from build123d import *

# Parameters (mm, degrees)
SKETCH1_W              = 16.002
SKETCH1_H              = 36.576
BOSS_EXTRUDE1_DEPTH    = 7.112
BOSS_EXTRUDE2_DEPTH    = 6.604
SKETCH3_W              = 16.002
SKETCH3_H              = 6.604
CUT_EXTRUDE1_DEPTH     = 2.54
SKETCH4_W              = 16.002
SKETCH4_H              = 2.54
CUT_EXTRUDE2_DEPTH     = 6.604
BOSS_EXTRUDE3_DEPTH    = 32.004
SKETCH6_W              = 32.004
SKETCH6_H              = 36.576
BOSS_EXTRUDE4_DEPTH    = 2.032
SKETCH7_W              = 16.002
SKETCH7_H              = 2.54
CUT_EXTRUDE3_DEPTH     = 6.604
M3_5_CLEARANCE_HOLE1_D = 3.7973


with BuildPart() as part:
    # Sketch1 → Boss-Extrude1 (new body)
    with BuildSketch(Plane(origin=(0, 7.874, 0), x_dir=(1, 0, 0), z_dir=(0, 1, 0))):
        with Locations((-8.001, 0)):
            Rectangle(SKETCH1_W, SKETCH1_H)
    extrude(amount=-BOSS_EXTRUDE1_DEPTH)

    # Sketch2 → Boss-Extrude2 (add)
    with BuildSketch(Plane.XZ.offset(-0.762)):
        with BuildLine():
            Line((-16.002, -18.288), (-16.002, 18.288))
            Line((-16.002, 18.288), (0, 18.288))
            Line((0, 18.288), (0, -15.748))
            add(Edge.make_bspline(
                [(0, -18.288), (0, -17.441333333), (0, -16.594666667), (0, -15.748)],
                knots=[0, 0, 0, 0, 1, 1, 1, 1], degree=3))
            Line((0, -18.288), (-16.002, -18.288))
        make_face()
    extrude(amount=BOSS_EXTRUDE2_DEPTH)

    # Sketch3 → Cut-Extrude1 (cut)
    with BuildSketch(Plane(origin=(0, 0, -18.288), x_dir=(-1, 0, 0), z_dir=(0, 0, -1))):
        with Locations((8.001, -2.54)):
            Rectangle(SKETCH3_W, SKETCH3_H)
    extrude(amount=-CUT_EXTRUDE1_DEPTH, mode=Mode.SUBTRACT)

    # Sketch4 → Cut-Extrude2 (cut)
    with BuildSketch(Plane.XZ.offset(5.842)):
        with Locations((-8.001, 17.018)):
            Rectangle(SKETCH4_W, SKETCH4_H)
    extrude(amount=-CUT_EXTRUDE2_DEPTH, mode=Mode.SUBTRACT)

    # Sketch5 → Boss-Extrude3 (add)
    with BuildSketch(Plane(origin=(0, 0, 0), x_dir=(0, 0, -1), z_dir=(1, 0, 0))):
        with BuildLine():
            Line((-18.288, -5.842), (-18.288, 0))
            ThreePointArc((-18.288, 0), (-12.964507707, 7.449482293), (-4.192296053, 4.826))
            Line((-4.192296053, 4.826), (4.192296053, 4.826))
            ThreePointArc((4.192296053, 4.826), (12.964507707, 7.449482293), (18.288, 0))
            Line((18.288, 0), (18.288, -5.842))
            Line((18.288, -5.842), (-18.288, -5.842))
        make_face()
        with BuildLine():
            Line((4.699, 0), (4.699, -5.715))
            Line((4.699, -5.715), (16.129, -5.715))
            Line((16.129, -5.715), (16.129, 0))
            ThreePointArc((16.129, 0), (10.414, 5.715), (4.699, 0))
        make_face(mode=Mode.SUBTRACT)
        with BuildLine():
            Line((-16.129, 0), (-16.129, -5.715))
            Line((-16.129, -5.715), (-4.699, -5.715))
            Line((-4.699, -5.715), (-4.699, 0))
            ThreePointArc((-4.699, 0), (-10.414, 5.715), (-16.129, 0))
        make_face(mode=Mode.SUBTRACT)
    extrude(amount=BOSS_EXTRUDE3_DEPTH)

    # Sketch6 → Boss-Extrude4 (add)
    with BuildSketch(Plane.XZ.offset(5.842)):
        with Locations((16.002, 0)):
            Rectangle(SKETCH6_W, SKETCH6_H)
    extrude(amount=BOSS_EXTRUDE4_DEPTH)

    # Sketch7 → Cut-Extrude3 (cut)
    with BuildSketch(Plane.XZ.offset(5.842)):
        with Locations((-8.001, 0)):
            Rectangle(SKETCH7_W, SKETCH7_H)
    extrude(amount=-CUT_EXTRUDE3_DEPTH, mode=Mode.SUBTRACT)

    # M3.5 Clearance Hole1 (through all)
    with Locations(Plane(origin=(0, 4.826, 0), x_dir=(1, 0, 0), z_dir=(0, 1, 0))):
        with Locations((25.654, 0), (6.604, 0)):
            Hole(M3_5_CLEARANCE_HOLE1_D / 2)


solid = part.part
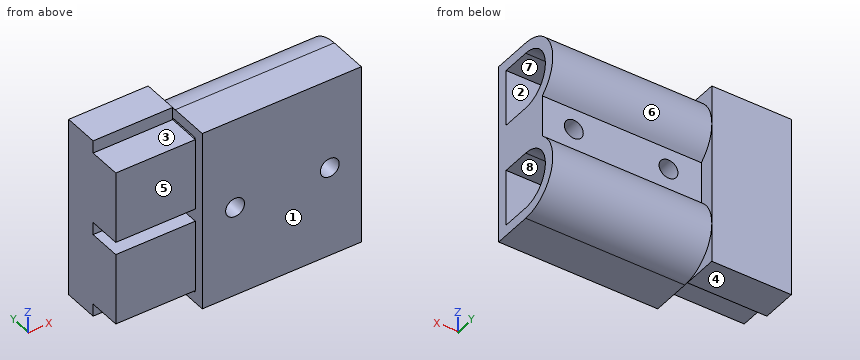
Verification items for the finished model (mm, model axes). Face numbers are marked on the shaded views. A direction names the side the tool comes from. Coordinates: 2 decimals unless noted, no trailing zeros. Write each loop counter-clockwise with the first axis right and the second up, starting at its lowest first coordinate (ties: lowest second). Pieces come first, ordered by that corner, then holes. Notation, with made-up numbers: M 69,-23.5 L 78,-23.5 A22 ccw 78,13.5 Z; hole C -5.75,65.25 d7. An arc over 180 degrees is marked long. Use a Markdown table: item, result.
Q1. Sectioned sample at B-B, the plane z = 0. Record the boundary of the cut face in (x, y), plus the area to 3 significant figures.
Reply:
| item | result |
|---|---|
| outline | M -16,0.76 L 0,0.76 L 0,-7.87 L 4.71,-7.87 L 4.71,4.83 L 0,4.83 L 0,7.87 L -16,7.87 Z; M 8.5,-7.87 L 23.76,-7.87 L 23.76,4.83 L 8.5,4.83 Z; M 27.55,-7.87 L 32,-7.87 L 32,4.83 L 27.55,4.83 Z |
| area | 424 mm² |
Q2. Draft check along Z on the marked faces 1, 2, 3 and 4. Enter one of: +Z half, -Z half, draft (parallel to the pull), parting line (faces both ways), or undercut.
Reply:
| item | result |
|---|---|
| face 1 | draft |
| face 2 | undercut |
| face 3 | +Z half |
| face 4 | -Z half |
Q3. Thickness scan on line 1 (Z direction, x = 14, y = -5.25); line 2 (Z direction, x = 13, y = 1.5); line 3 (Z direction, x = -9, y = -4). Record the ranges inside material, lowest first.
Reply:
| item | result |
|---|---|
| line 1 | z = -18.29 to -16.13, -4.7 to 4.7, 16.13 to 18.29 |
| line 2 | z = -18.14 to -15.93, -4.9 to 4.9, 15.93 to 18.14 |
| line 3 | z = -15.75 to -1.27, 1.27 to 15.75 |
Q4. Set-up check for the marked faces 5, 6, 7 and 8: record each of +Z, -Z, +X, -X, +Y, -Y from which the full face is reachable in a straight line by a thin tool's end or side.
Reply:
| item | result |
|---|---|
| face 5 | +Z, -Z, -X, -Y |
| face 6 | +X, +Y |
| face 7 | +X, -X |
| face 8 | +X |
Q5. Go/stop test with flat-tipped pins: P1, Ø2, axis at x = -4.5, z = -0.5, coming from the -Y side; P2, Ø5.5, axis at x = -9, y = -1, coming from the +Z side; P3, Ø9, axis at x = 19, z = -0.5, coming from the +Y side; P4, Ø2, axis at x = 10, y = 2.5, coming from the -Z side. Record where each tip stops, or that it passes through.
Reply:
| item | result |
|---|---|
| P1 | stops at y = -5.84 |
| P2 | stops at z = 18.29 |
| P3 | stops at y = 5.72 |
| P4 | stops at z = -18.14 |
Q6. Sectioned sample at C-C, the plane x = 23. Record the boundary of the cut face in (y, z) (3 decimals).
Reply:
| item | result |
|---|---|
| outline | M -7.874,-18.288 L 0,-18.288 A7.874 ccw 4.826,-4.192 L 4.826,4.192 A7.874 ccw 0,18.288 L -7.874,18.288 Z; hole M -5.715,-16.129 L 0,-16.129 A5.715 ccw 0,-4.699 L -5.715,-4.699 Z; hole M -5.715,4.699 L 0,4.699 A5.715 ccw 0,16.129 L -5.715,16.129 Z |
Q7. Sectioned sample at A-A, the plane x = 7.5. Record the boundary of the cut face in (y, z) (3 decimals).
Reply:
| item | result |
|---|---|
| outline | M -7.874,-18.288 L 0,-18.288 A7.874 ccw 4.826,-4.192 L 4.826,-1.674 L -7.874,-1.674 Z; M -7.874,1.674 L 4.826,1.674 L 4.826,4.192 A7.874 ccw 0,18.288 L -7.874,18.288 Z; hole M -5.715,-16.129 L 0,-16.129 A5.715 ccw 0,-4.699 L -5.715,-4.699 Z; hole M -5.715,4.699 L 0,4.699 A5.715 ccw 0,16.129 L -5.715,16.129 Z |
Q8. Sectioned sample at D-D, the plane z = 8. Record the boundary of the cut face in (x, y) (3 decimals), plus the area to 3 significant figures.
Reply:
| item | result |
|---|---|
| outline | M -16.002,-5.842 L 0,-5.842 L 0,-7.874 L 32.004,-7.874 L 32.004,-5.715 L 0,-5.715 L 0,5.18 L 32.004,5.18 L 32.004,7.495 L 0,7.495 L 0,7.874 L -16.002,7.874 Z |
| area | 363 mm² |
